from build123d import *

# Parameters (mm, degrees)
SKETCH1_W               = 22
SKETCH1_H               = 10
BOSS_EXTRUDE1_DEPTH     = 25
FILLET1_R               = 5
FILLET2_R               = 5
FILLET3_R               = 5
FILLET4_R               = 5
FILLET5_R               = 2
FILLET6_R               = 1
FILLET7_R               = 3
FILLET8_R               = 5
CUT_EXTRUDE1_DEPTH      = 35
CUT_EXTRUDE1_DEPTH_BACK = 25
SKETCH2_W               = 5.25
SKETCH2_H               = 2
BOSS_EXTRUDE2_DEPTH     = 25
FILLET9_R               = 1


# Some blends are built 0.0001 mm under size
with BuildPart() as part:
    # Sketch1 → Boss-Extrude1 (new body)
    with BuildSketch(Plane(origin=(0, 0, 0), x_dir=(0, 0, -1), z_dir=(1, 0, 0))):
        with BuildLine():
            ThreePointArc((-15.5, -17.5), (-55.5, -57.5), (-15.5, -97.5))
            Line((-15.5, -97.5), (19.5, -97.5))
            Line((19.5, -97.5), (19.5, -117.5))
            Line((19.5, -117.5), (-15.5, -117.5))
            ThreePointArc((-15.5, -117.5), (-75.455538985, -59.809403615), (-20.115384615, 2.322221831))
            Line((-20.115384615, 2.322221831), (-15.115384615, 32.514814847))
            Line((-15.115384615, 32.514814847), (-10.115384615, 32.514814847))
            Line((-10.115384615, 32.514814847), (-10.115384615, 7.5))
            Line((-10.115384615, 7.5), (10.884615385, 7.5))
            Line((10.884615385, 7.5), (10.884615385, 32.514814847))
            Line((10.884615385, 32.514814847), (15.884615385, 32.514814847))
            Line((15.884615385, 32.514814847), (20.8, -2.5))
            Line((20.8, -2.5), (0, -17.5))
            Line((0, -17.5), (-15.5, -17.5))
        make_face()
        with BuildLine():
            ThreePointArc((-52.30218335, -98.372965401), (-35.210237225, -108.846923457), (-15.5, -112.5))
            Line((-15.5, -112.5), (-15.5, -102.5))
            ThreePointArc((-15.5, -102.5), (-31.62655773, -99.511119192), (-45.610877286, -90.941517146))
            Line((-45.610877286, -90.941517146), (-52.30218335, -98.372965401))
        make_face(mode=Mode.SUBTRACT)
        with BuildLine():
            ThreePointArc((-56.372965401, -20.69781665), (-66.313374288, -36.45241122), (-70.424624412, -54.621522407))
            Line((-70.424624412, -54.621522407), (-60.438329064, -55.144881969))
            ThreePointArc((-60.438329064, -55.144881969), (-57.074578963, -40.279245544), (-48.941517146, -27.389122714))
            Line((-48.941517146, -27.389122714), (-56.372965401, -20.69781665))
        make_face(mode=Mode.SUBTRACT)
        with BuildLine():
            ThreePointArc((-21.24906548, -2.801295755), (-37.870515369, -7.25499983), (-52.30218335, -16.627034599))
            Line((-52.30218335, -16.627034599), (-45.610877286, -24.058482854))
            ThreePointArc((-45.610877286, -24.058482854), (-33.803148938, -16.390454406), (-20.203780847, -12.746514708))
            Line((-20.203780847, -12.746514708), (-21.24906548, -2.801295755))
        make_face(mode=Mode.SUBTRACT)
        Polygon((8.463652775, -2.5), (-7.917479229, -12.773905232), (-10.115384615, -12.773905232), (-10.115384615, -2.5), align=None, mode=Mode.SUBTRACT)
        with Locations((1.5, -107.5)):
            Rectangle(SKETCH1_W, SKETCH1_H, mode=Mode.SUBTRACT)
        with BuildLine():
            Line((-60.438329064, -59.855118031), (-70.424624412, -60.378477593))
            ThreePointArc((-70.424624412, -60.378477593), (-66.313374288, -78.54758878), (-56.372965401, -94.30218335))
            Line((-56.372965401, -94.30218335), (-48.941517146, -87.610877286))
            ThreePointArc((-48.941517146, -87.610877286), (-57.074578963, -74.720754456), (-60.438329064, -59.855118031))
        make_face(mode=Mode.SUBTRACT)
    extrude(amount=-BOSS_EXTRUDE1_DEPTH)

    # Fillet1
    fillet1_edges = [part.edges().sort_by_distance(p)[0] for p in [
        (-12.5, -90.941517146, 45.610877286),
        (-12.5, -102.5, 9.5),
        (-12.5, -112.5, 9.5),
        (-12.5, -112.5, 15.5),
        (-12.5, -112.5, -12.5),
        (-12.5, -102.5, -12.5),
        (-12.5, -98.372965401, 52.30218335),
        (-12.5, -102.5, 15.5),
        (-12.5, -87.610877286, 48.941517146),
        (-12.5, -94.30218335, 56.372965401),
        (-12.5, -20.69781665, 56.372965401),
        (-12.5, -27.389122714, 48.941517146),
        (-12.5, -55.144881969, 60.438329064),
        (-12.5, -54.621522407, 70.424624412),
        (-12.5, -16.627034599, 52.30218335),
        (-12.5, -24.058482854, 45.610877286),
        (-12.5, -12.746514708, 20.203780847),
        (-12.5, -2.801295755, 21.24906548),
    ]]
    fillet(fillet1_edges, radius=FILLET1_R - 0.0001)  # a hair under: the kernel refuses the full size

    # Fillet2
    fillet2_edges = [part.edges().sort_by_distance(p)[0] for p in [
        (-12.5, -59.855118031, 60.438329064),
        (-12.5, -60.378477593, 70.424624412),
    ]]
    fillet(fillet2_edges, radius=FILLET2_R - 0.0001)  # a hair under: the kernel refuses the full size

    # Fillet3
    fillet3_edges = [part.edges().sort_by_distance(p)[0] for p in [
        (-12.5, -2.5, 10.115384615),
    ]]
    fillet(fillet3_edges, radius=FILLET3_R)

    # Fillet4
    # the kernel refuses this fillet: 5 mm, written as the material it adds along each edge
    with BuildSketch(Plane(origin=(0, -12.773905232, 10.115384615), x_dir=(0, 1, 0), z_dir=(-1, 0, 0))) as fillet4_piece_1:
        with BuildLine():
            CenterArc((4.141046459, 5), FILLET4_R, 214.08477399, 55.91522601)
            Line((0, 2.197905387), (-0.082820929, 2.141863494))
            ThreePointArc((-0.082820929, 2.141863494), (-0.1, 1.098952693), (-0.1, 0))
            Line((-0.1, 0), (0, -0.1))
            Line((0, -0.1), (4.141046459, -0.1))
            Line((4.141046459, -0.1), (4.141046459, 0))
        make_face()
    extrude(amount=25)

    # Fillet5
    fillet5_edges = [part.edges().sort_by_distance(p)[0] for p in [
        (-12.5, -12.773905232, 7.917479229),
    ]]
    fillet(fillet5_edges, radius=FILLET5_R)

    # Fillet6
    fillet6_edges = [part.edges().sort_by_distance(p)[0] for p in [
        (-12.5, -2.5, -8.463652775),
    ]]
    fillet(fillet6_edges, radius=FILLET6_R)

    # Fillet7
    fillet7_edges = [part.edges().sort_by_distance(p)[0] for p in [
        (-12.5, 2.322221831, 20.115384615),
        (-12.5, -2.5, -20.8),
        (-12.5, -17.5, 0),
    ]]
    fillet(fillet7_edges, radius=FILLET7_R)

    # Fillet8
    fillet8_edges = [part.edges().sort_by_distance(p)[0] for p in [
        (-12.5, -97.5, -19.5),
        (-12.5, -117.5, -19.5),
    ]]
    fillet(fillet8_edges, radius=FILLET8_R)

    # Sketch2 → Cut-Extrude1 (cut, two sides: drawn at the far end of the back side and taken through both)
    with BuildSketch(Plane.XY.offset(-10.884615385).offset(-CUT_EXTRUDE1_DEPTH_BACK)):
        with Locations((-17.375, 29)):
            Rectangle(SKETCH2_W, SKETCH2_H)
        with Locations((-7.625, 29)):
            Rectangle(SKETCH2_W, SKETCH2_H)
    extrude(amount=CUT_EXTRUDE1_DEPTH + CUT_EXTRUDE1_DEPTH_BACK, mode=Mode.SUBTRACT)

    # Sketch3 → Boss-Extrude2 (add)
    with BuildSketch(Plane(origin=(0, 0, 0), x_dir=(0, 0, -1), z_dir=(1, 0, 0))):
        Polygon((16.937466436, 25.014814847), (18.937466436, 25.295575128), (15.884615385, 32.514814847), align=None)
        Polygon((-16.357411095, 25.014814847), (-18.357411095, 25.346021908), (-15.115384615, 32.514814847), align=None)
    extrude(amount=-BOSS_EXTRUDE2_DEPTH)

    # Fillet9
    fillet9_edges = [part.edges().sort_by_distance(p)[0] for p in [
        (-12.5, 25.295575128, -18.937466436),
        (-12.5, 25.346021908, 18.357411095),
    ]]
    fillet(fillet9_edges, radius=FILLET9_R)


solid = part.part
The listing builds one solid part. Answer for the finished solid, in the listing's coordinates (mm). A direction names the side the tool comes from. Round coordinates to 2 decimals unless told otherwise and drop trailing zeros. Write each loop counter-clockwise with the first axis right and the second up, starting at its lowest first coordinate (ties: lowest second). Pieces come first, ordered by that corner, then holes. Notation, with made-up numbers: (39, 39.5) - (82, 39.5) arc R23 ccw to (82, 63.5) - close; hole circle Ø5 at (-13.5, 60.5). An arc over 180 degrees is marked (long way). Use one line per item in the form item = value. Start each with the question number.
Item 1: A cutting plane is placed at C-C (x = -6.5). Give the number of separate pieces and of enclosed holes in the cut face, plus the area to 3 significant figures.
Item 2: Find the intervals of material crossed by line 1 (Y direction, x = -18, z = 13.5); line 2 (Y direction, x = -8, z = 31); line 3 (Y direction, x = -18.5, z = -12), in increasing order. Write a range as [from, to].
Item 3: Determine the mould class of faces 4 (the flat face through (-17, 30, -14)), 5 (the flat face through (-12, 32.515, 13)), 6 (the cylindrical face through (-12.68, -116, -18.07)) for opening direction Y: +Y half, -Y half, draft (parallel to the pull), parting line (faces both ways), or undercut.
Item 4: A cutting plane is placed at B-B (y = 9.5). Write down the section's boundary in (x, z).
Item 5: A cutting plane is placed at D-D (y = -78.5). Write down the section's boundary in (x, z).
Item 6: A cutting plane is placed at A-A (z = 12). Write down the section's boundary in (x, y), plus the area to 3 significant figures.
Item 7: Flat-ended cylindrical pins translate along their axes: pin 1 Ø8 at (x, z) = (-21, 51) entering from +Y; pin 2 Ø1.5 at (x, y) = (-7, -67) entering from -Z; pin 3 Ø10.5 at (x, z) = (-6.5, 3) entering from +Y. Find the tip coordinate at first contact, or state that the pin passes through.
Item 8: A tool of negligible diameter and unlimited length cuts with its end or side. For faces 1 (the cylindrical face through (-12.325, -78.377, 66.384)), 2 (the flat face through (-12.325, 14.663, 18.072)), 3 (the flat face through (-8, 30, 13)), from which of +Z, -Z, +X, -X, +Y, -Y can it reach the whole face along a straight path? Write none if from no direction.
The answers:
q1.separate_pieces = 1
q1.enclosed_holes = 6
q1.area = 3,370 mm^2
q2.line_1 = [-117.5, -97.5], [-17.5, 28], [30, 32.51]
q2.line_2 = [-115.46, -110.27], [-99.75, -94.37], [-20.63, -15.25], [-4.73, 0.46]
q2.line_3 = [-117.5, -109.68], [-105.32, -97.5], [-8.85, 28], [30, 32.51]
q3.face_4 = undercut
q3.face_5 = +Y half
q3.face_6 = -Y half
q4.outline = (-25, -19.12) - (0, -19.12) - (0, -10.88) - (-25, -10.88) - close; (-25, 10.12) - (0, 10.12) - (0, 18.93) - (-25, 18.93) - close
q5.outline = (-25, 49.54) - (0, 49.54) - (0, 55.3) - (-25, 55.3) - close; (-25, 66.33) - (0, 66.33) - (0, 71.7) - (-25, 71.7) - close
q6.outline = (-25, -117.5) - (0, -117.5) - (0, -97.5) - (-25, -97.5) - close; (-25, -17.5) - (0, -17.5) - (0, 32.51) - (-25, 32.51) - close; hole (-20, 28) - (-14.75, 28) - (-14.75, 30) - (-20, 30) - close; hole (-10.25, 28) - (-5, 28) - (-5, 30) - (-10.25, 30) - close
q6.area = 1,730 mm^2
q7.pin_1 = -6.43
q7.pin_2 = 54.16
q7.pin_3 = 7.5
q8.face_1 = +X, -X
q8.face_2 = +Z, +X, -X
q8.face_3 = none
